Here's how the part is built. I have some questions about the finished solid (model axes, mm). Coordinates: 2 decimals unless noted, no trailing zeros. Write each loop counter-clockwise with the first axis right and the second up, starting at its lowest first coordinate (ties: lowest second). Pieces come first, ordered by that corner, then holes. Notation, with made-up numbers: (-20.5, -39.75) -> (9.5, -39.75) arc R30 ccw to (9.5, -4.75) -> close; hole circle Ø10 at (-38, 73). An arc over 180 degrees is marked (long way). Use a Markdown table: item, result. Add a question column.
Item 1: If I drill on line 1 along X through (y, z) = (6.5, 0); line 2 along X through (y, z) = (2.5, -23.5); line 3 along Z through (x, y) = (-35, 6), over which ranges is the centre line in solid material (lowest first)? Write a range as from..to.
Item 2: Imagine slicing it at B-B, the plane x = -2. Write out the boundary of the cut face in (y, z), and give its area (3 significant figures).
Item 3: Imagine slicing it at C-C, the plane y = 3.25. Write out the boundary of the cut face in (x, z), and give its area (3 significant figures).
Item 4: Will this pin go through, and if not, where does the flat tip stop? pin 1 Ø1.8 at (x, z) = (35, -23.5) entering from -Y.
Item 5: Imagine slicing it at A-A, the plane z = 0. Write out the boundary of the cut face in (x, y), and give its area (3 significant figures).
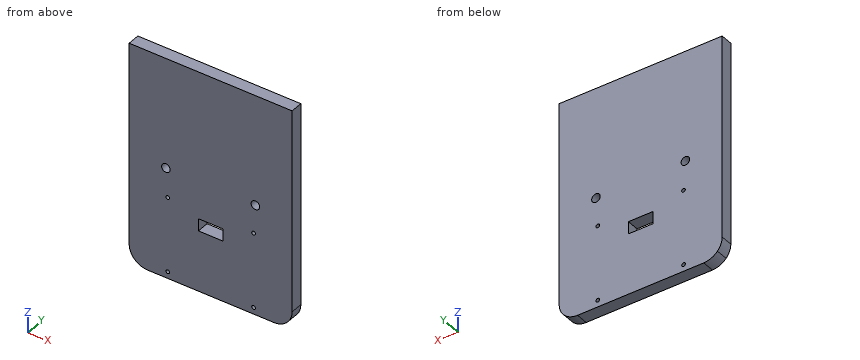
```python
from build123d import *

# Parameters (mm, degrees)
SKETCH1_R           = 3.5
SKETCH1_R_2         = 1.5
SKETCH1_W           = 20
SKETCH1_H           = 10
BOSS_EXTRUDE1_DEPTH = 10


with BuildPart() as part:
    # Sketch1 → Boss-Extrude1 (new body)
    with BuildSketch(Plane(origin=(0, 0, 0), x_dir=(1, 0, 0), z_dir=(0, 1, 0))):
        Polygon((0.049612108, 0.067144207), (-66.5, -90), (66.5, -90), align=None)
        with BuildLine():
            Line((-66.5, 75), (-66.5, -90))
            Line((-66.5, -90), (0.049612108, 0.067144207))
            Line((0.049612108, 0.067144207), (-62.643246745, 85.041317243))
            ThreePointArc((-62.643246745, 85.041317243), (-65.502655126, 80.378257098), (-66.5, 75))
        make_face()
        with Locations((-36.5, 0)):
            Circle(SKETCH1_R, mode=Mode.SUBTRACT)
        with Locations((-35, 23.5)):
            Circle(SKETCH1_R_2, mode=Mode.SUBTRACT)
        with BuildLine():
            Line((62.748695437, 84.923046456), (0.049612108, 0.067144207))
            Line((0.049612108, 0.067144207), (66.5, -90))
            Line((66.5, -90), (66.5, 75))
            ThreePointArc((66.5, 75), (65.530866537, 80.304223244), (62.748695437, 84.923046456))
        make_face()
        with Locations((36.5, 0)):
            Circle(SKETCH1_R, mode=Mode.SUBTRACT)
        with Locations((35, 23.5)):
            Circle(SKETCH1_R_2, mode=Mode.SUBTRACT)
        with BuildLine():
            Line((-62.643246745, 85.041317243), (0.049612108, 0.067144207))
            Line((0.049612108, 0.067144207), (62.748695437, 84.923046456))
            ThreePointArc((62.748695437, 84.923046456), (57.670668649, 88.671973099), (51.5, 90))
            Line((51.5, 90), (-51.5, 90))
            ThreePointArc((-51.5, 90), (-57.598370329, 88.704374459), (-62.643246745, 85.041317243))
        make_face()
        with Locations((-35, 84.5)):
            Circle(SKETCH1_R_2, mode=Mode.SUBTRACT)
        with Locations((0, 35.5)):
            Rectangle(SKETCH1_W, SKETCH1_H, mode=Mode.SUBTRACT)
        with Locations((35, 84.5)):
            Circle(SKETCH1_R_2, mode=Mode.SUBTRACT)
    extrude(amount=BOSS_EXTRUDE1_DEPTH)


solid = part.part
```
Ans:
| question | item | result |
|---|---|---|
| 1 | line 1 | x = -66.5..-40, -33..33, 40..66.5 |
| 1 | line 2 | x = -66.5..-36.5, -33.5..33.5, 36.5..66.5 |
| 1 | line 3 | z = -90..-86, -83..-25, -22..-3.16, 3.16..90 |
| 2 | outline | (0, -90) -> (10, -90) -> (10, -40.5) -> (0, -40.5) -> close; (0, -30.5) -> (10, -30.5) -> (10, 90) -> (0, 90) -> close |
| 2 | area | 1,700 mm^2 |
| 3 | outline | (-66.5, -75) arc R15 ccw to (-51.5, -90) -> (51.5, -90) arc R15 ccw to (66.5, -75) -> (66.5, 90) -> (-66.5, 90) -> close; hole circle Ø7 at (-36.5, 0); hole circle Ø3 at (-35, -84.5); hole circle Ø3 at (-35, -23.5); hole (-10, -40.5) -> (10, -40.5) -> (10, -30.5) -> (-10, -30.5) -> close; hole circle Ø7 at (36.5, 0); hole circle Ø3 at (35, -84.5); hole circle Ø3 at (35, -23.5) |
| 3 | area | 23,500 mm^2 |
| 4 | pin 1 | passes through |
| 5 | outline | (-66.5, 0) -> (-40, 0) -> (-40, 10) -> (-66.5, 10) -> close; (-33, 0) -> (33, 0) -> (33, 10) -> (-33, 10) -> close; (40, 0) -> (66.5, 0) -> (66.5, 10) -> (40, 10) -> close |
| 5 | area | 1,190 mm^2 |
